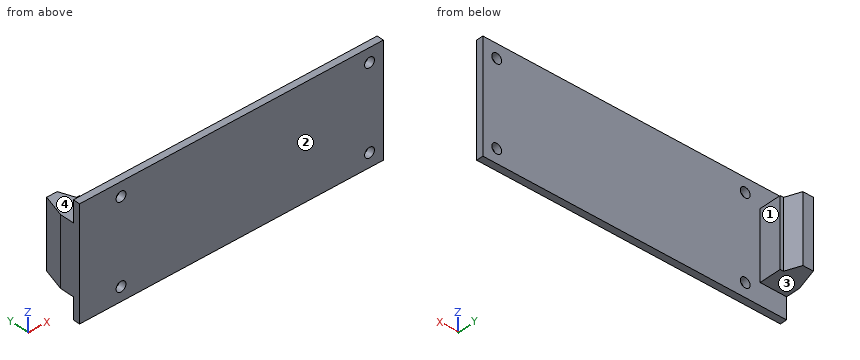
```python
from build123d import *

# Parameters (mm, degrees)
SKETCH2_W                 = 69.85
SKETCH2_H                 = 25.4
BOSS_EXTRUDE1_DEPTH       = 1.5748
TAP_DRILL_FOR_4_40_TAP1_D = 2.2606
BOSS_EXTRUDE2_DEPTH       = 7.8105


with BuildPart() as part:
    # Sketch2 → Boss-Extrude1 (new body)
    with BuildSketch(Plane(origin=(0, 0, 0), x_dir=(1, 0, 0), z_dir=(0, 1, 0))):
        with Locations((34.925, 12.7)):
            Rectangle(SKETCH2_W, SKETCH2_H)
    extrude(amount=BOSS_EXTRUDE1_DEPTH)

    # Tap Drill for #4-40 Tap1 (through all)
    with Locations(Plane(origin=(9.525, 1.5748, -22.225), x_dir=(0, 0, 1), z_dir=(0, 1, 0))):
        with Locations((0, 0), (19.05, 0), (19.05, 57.15), (0, 57.15)):
            Hole(TAP_DRILL_FOR_4_40_TAP1_D / 2)

    # Sketch4 → Boss-Extrude2 (add, symmetric)
    with BuildSketch(Plane.XY.offset(-12.7)):
        Polygon((0, 1.5748), (0, 4.817906029), (1.588475565, 10.0838), (3.999524435, 10.0838), (5.314976691, 6.6548), (6.096, 6.6548), (6.096, 1.5748), align=None)
    extrude(amount=BOSS_EXTRUDE2_DEPTH, both=True)


solid = part.part
```
Source: CAD feature listing. Evaluate the final solid. Frame: model axes, mm. Face numbers are marked on the shaded views. A direction names the side the tool comes from. Give positions to 0.01 mm unless a question says otherwise; leave off trailing zeros. Loops run counter-clockwise (first coordinate to the right, second up) from the corner with the lowest first, then second, coordinate; pieces in that order, holes last. Notation, with made-up numbers: (28.5, 88) - (40.5, 88) arc R14 cw to (40.5, 92) - close; hole circle Ø7 at (46, -10). An arc over 180 degrees is marked (long way). Use CSV: the item, a comma, the result in double quotes.
1) Line query: line 1 (X direction, y = 1.5, z = -3); line 2 (Y direction, x = 67.5, z = -19); line 3 (X direction, y = 1.5, z = -23). Output: solid intervals per line, ascending.
Worked out:
line 1,"x = 0 to 8.41, 10.64 to 65.56, 67.79 to 69.85"
line 2,"y = 0 to 1.57"
line 3,"x = 0 to 8.7, 10.35 to 65.85, 67.5 to 69.85"
2) Cut plane C-C (x = 56). Output: boundary loops of the cut face in (y, z), and give its area (3 significant figures).
Worked out:
outline,"(0, -25.4) - (1.57, -25.4) - (1.57, 0) - (0, 0) - close"
area,"40.0 mm^2"
3) Cut plane A-A (z = -22.5). Output: boundary loops of the cut face in (x, y).
Worked out:
outline,"(0, 0) - (8.43, 0) - (8.43, 1.57) - (0, 1.57) - close; (10.62, 0) - (65.58, 0) - (65.58, 1.57) - (10.62, 1.57) - close; (67.77, 0) - (69.85, 0) - (69.85, 1.57) - (67.77, 1.57) - close"
4) Set-up query: the marked faces 1, 2, 3 and 4. Return all of +Z, -Z, +X, -X, +Y, -Y with unobstructed straight access to the full face (end or side cutting, diameter ignored); none if empty.
Worked out:
face 1,"+Z, -Z, +X, +Y"
face 2,"+Z, -Z, +X, -X, -Y"
face 3,"-Z, +X, -X, +Y"
face 4,"+Z, +X, -X, +Y"
5) Pin query (flat end, axial travel): P1, Ø7.5, axis at x = 17.5, z = -13.5, coming from the +Y side; P2, Ø1.4, axis at x = 9.525, z = -22.225, coming from the -Y side; P3, Ø1.5, axis at y = 5, z = -15.5, coming from the +X side; P4, Ø1.8, axis at x = 4, y = 6.5, coming from the -Z side. Return the tip coordinate at first contact, or that it passes through.
Worked out:
P1,"stops at y = 1.57"
P2,"passes through"
P3,"stops at x = 6.1"
P4,"stops at z = -20.51"
6) Cut plane D-D (y = 2.25). Output: boundary loops of the cut face in (x, z), and give its area (3 significant figures).
Worked out:
outline,"(0, -20.51) - (6.1, -20.51) - (6.1, -4.89) - (0, -4.89) - close"
area,"95.2 mm^2"
7) Cut plane B-B (z = -12). Output: boundary loops of the cut face in (x, y).
Worked out:
outline,"(0, 0) - (69.85, 0) - (69.85, 1.57) - (6.1, 1.57) - (6.1, 6.65) - (5.31, 6.65) - (4, 10.08) - (1.59, 10.08) - (0, 4.82) - close"
